Input: part model. Units: mm. Frame: model coordinates. Face numbers are marked on the shaded views. A direction names the side the tool comes from. Coordinates: 2 decimals unless noted, no trailing zeros. Order: outer loops, then holes, each group sorted by start corner. A loop starts at its lowest first (then second) coordinate and runs counter-clockwise, first axis right, second up. Notation, with made-up numbers: (48.5, 65) - (102.5, 65) arc R21 ccw to (102.5, 84) - close; hole circle Ø9 at (66.25, 71.5). An arc over 180 degrees is marked (long way). One line per question, with ' | ' between items.
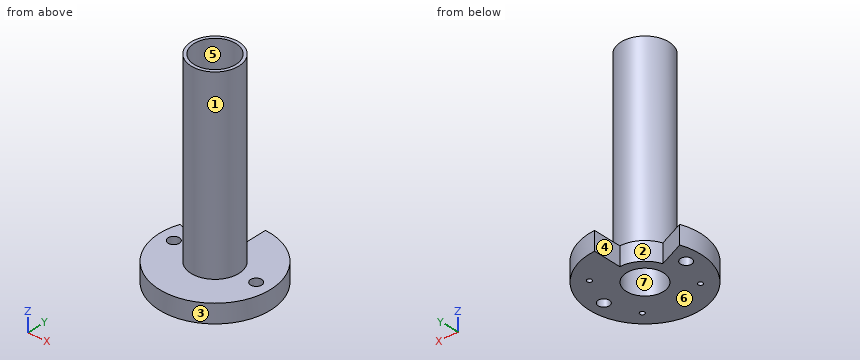
from build123d import *

# Parameters (mm, degrees)
SKETCH1_R                 = 30
BOSS_EXTRUDE1_DEPTH       = 10
SKETCH2_R                 = 12.9
BOSS_EXTRUDE2_DEPTH       = 50
F_6_0MM_DOWEL_HOLE1_D     = 6
CUT_EXTRUDE2_START        = -50
CUT_EXTRUDE2_DEPTH        = 50
F_2_5MM_DOWEL_HOLE1_D     = 2.5
F_2_5MM_DOWEL_HOLE1_DEPTH = 5
SKETCH15_R                = 12.9
SKETCH15_R_2              = 11.25
BOSS_EXTRUDE3_DEPTH       = 50
F_6_0MM_DOWEL_HOLE2_D     = 20


with BuildPart() as part:
    # Sketch1 → Boss-Extrude1 (new body)
    with BuildSketch(Plane.XY):
        Circle(SKETCH1_R)
    extrude(amount=BOSS_EXTRUDE1_DEPTH)

    # Sketch2 → Boss-Extrude2 (add)
    with BuildSketch(Plane.XY.offset(10)):
        Circle(SKETCH2_R)
    extrude(amount=BOSS_EXTRUDE2_DEPTH)

    # Ø6.0mm Dowel Hole1 (through all)
    with Locations(Plane.XY.offset(10)):
        with Locations((-22.25, 0), (22.25, 0)):
            Hole(F_6_0MM_DOWEL_HOLE1_D / 2)

    # Sketch7 → Cut-Extrude2 (cut)
    with BuildSketch(Plane.XY.offset(10).offset(CUT_EXTRUDE2_START)):
        with BuildLine():
            Line((0, 15), (0, 30))
            ThreePointArc((0, 30), (-17.161157118, 24.606801628), (-28.152079261, 10.366312424))
            Line((-28.152079261, 10.366312424), (-14.149156244, 4.98009815))
            ThreePointArc((-14.149156244, 4.98009815), (-8.668867508, 12.241353525), (0, 15))
        make_face()
    extrude(amount=CUT_EXTRUDE2_DEPTH, mode=Mode.SUBTRACT)

    # Ø2.5mm Dowel Hole1
    with Locations(Plane(origin=(0, 0, 0), x_dir=(-1, 0, 0), z_dir=(0, 0, -1))):
        with Locations((-15.733125881, 15.733125881), (-15.733125881, -15.733125881), (15.733125881, -15.733125881)):
            Hole(F_2_5MM_DOWEL_HOLE1_D / 2, depth=F_2_5MM_DOWEL_HOLE1_DEPTH)

    # Sketch15 → Boss-Extrude3 (add)
    with BuildSketch(Plane.XY.offset(60)):
        Circle(SKETCH15_R)
        Circle(SKETCH15_R_2, mode=Mode.SUBTRACT)
    extrude(amount=BOSS_EXTRUDE3_DEPTH)

    # Ø6.0mm Dowel Hole2 (through all)
    with Locations(Plane(origin=(0, 0, 0), x_dir=(-1, 0, 0), z_dir=(0, 0, -1))):
        with Locations((0, 0)):
            Hole(F_6_0MM_DOWEL_HOLE2_D / 2)


solid = part.part
Item 1: Section C-C on z = 99.5. Return the cut outline in (x, y).
Data:
outline: circle Ø25.8 at (0, 0); hole circle Ø22.5 at (0, 0)
Item 2: Ray query, line 1 (Y direction, x = 0, z = 95); line 2 (X direction, y = -0.5, z = 28.5); line 3 (Y direction, x = 0, z = 45.5). Return the intervals inside material, ascending.
Data:
line 1: -12.9 to -11.25, 11.25 to 12.9 | line 2: -12.89 to -9.99, 9.99 to 12.89 | line 3: -12.9 to -10, 10 to 12.9
Item 3: Section A-A on y = 0. Return the cut outline in (x, z), and give its area (3 significant figures).
Data:
outline: (-30, 0) - (-25.25, 0) - (-25.25, 10) - (-30, 10) - close; (-19.25, 0) - (-10, 0) - (-10, 60) - (-11.25, 60) - (-11.25, 110) - (-12.9, 110) - (-12.9, 10) - (-19.25, 10) - close; (10, 0) - (19.25, 0) - (19.25, 10) - (12.9, 10) - (12.9, 110) - (11.25, 110) - (11.25, 60) - (10, 60) - close; (25.25, 0) - (30, 0) - (30, 10) - (25.25, 10) - close | area: 735 mm^2
Item 4: Section B-B on x = -20.5. Return the cut outline in (y, z), and give its area (3 significant figures).
Data:
outline: (-21.9, 0) - (-2.44, 0) - (-2.44, 10) - (-21.9, 10) - close; (2.44, 0) - (7.42, 0) - (7.42, 10) - (2.44, 10) - close | area: 245 mm^2
Item 5: Contact query for flat-ended pins moving along their axis: P1, Ø2, axis at x = -15.73, y = -15.73, coming from the -Z side; P2, Ø2, axis at x = 13, y = 22.5, coming from the +Z side; P3, Ø8, axis at y = 19.5, z = 6.5, coming from the -X side. Output: stop coordinate, or through.
Data:
P1: z = 5 | P2: z = 10 | P3: x = 0
Item 6: Section D-D on x = 22.25. Return the cut outline in (y, z).
Data:
outline: (-20.12, 0) - (-3, 0) - (-3, 10) - (-20.12, 10) - close; (3, 0) - (20.12, 0) - (20.12, 10) - (3, 10) - close
Item 7: Access query for the marked faces 1, 2 and 3. Directions: +Z, -Z, +X, -X, +Y, -Y. A direction counts if a zero-diameter tool reaches every point of the face in a straight line with its end or side. Return the directions, or none.
Data:
face 1: +Z | face 2: +Z, -Z, +Y | face 3: +Z, -Z
Item 8: Draft query along X for the marked faces 4, 5, 6 and 7. Return one class per face: released by +X, released by -X, zero draft, split by the parting line, or undercut.
Data:
face 4: released by -X | face 5: undercut | face 6: zero draft | face 7: undercut
